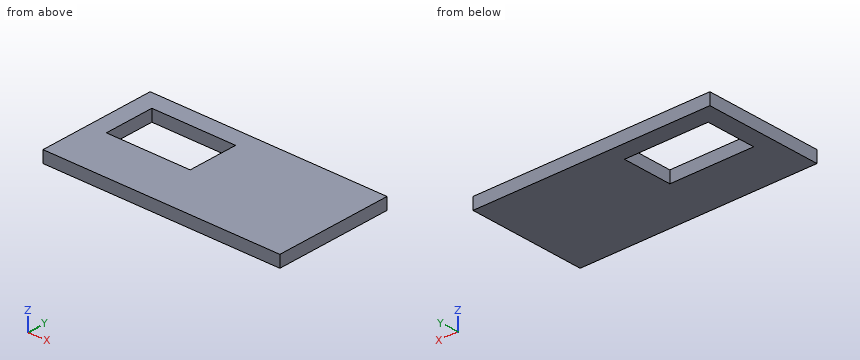
```python
from build123d import *

# Parameters (mm, degrees)
F0_W     = 200
F0_H     = 100
F1_DEPTH = 10
F3_DEPTH = 25


with BuildPart() as f1:
    # F0 (on Top) → F1 (new body)
    with BuildSketch(Plane.XY):
        with Locations((8.938173, -34.933871)):
            Rectangle(F0_W, F0_H)
    extrude(amount=F1_DEPTH)

    # F2 (on face) → F3 (cut)
    with BuildSketch(Plane.XY.offset(10)):
        Polygon((-5.306835, -42.385153), (-5.306835, 0), (-76.061827, 0.066129), (-76.061827, -42.385153), align=None)
    extrude(amount=-F3_DEPTH, mode=Mode.SUBTRACT)


solid = f1.part
```
Verification items for the finished model (mm, model axes). Give positions to 0.01 mm unless a question says otherwise; leave off trailing zeros. Order: outer loops, then holes, each group sorted by start corner. A loop starts at its lowest first (then second) coordinate and runs counter-clockwise, first axis right, second up. Notation, with made-up numbers: (43, -3.75) - (56, -3.75) arc R27 ccw to (56, 17.25) - close; hole circle Ø7 at (31, -35). An arc over 180 degrees is marked (long way). Answer as CSV lines item,"result". Start each with the question number.
Item 1: Section check C-C, the plane x = -46. Record the boundary of the cut face in (y, z).
Item 2: Material ranges on L1, parallel to X at y = -12, z = 8.25; L2, parallel to Y at x = -10, z = 4; L3, parallel to Y at x = -60.5, z = 4.5, recorded low to high.
Item 3: Section check A-A, the plane y = -39.5. Record the boundary of the cut face in (x, z), plus the area to 3 significant figures.
Item 4: Section check B-B, the plane z = 4.5. Record the boundary of the cut face in (x, y), plus the area to 3 significant figures.
Filled in:
1,outline,"(-84.93, 0) - (-42.39, 0) - (-42.39, 10) - (-84.93, 10) - close; (0.04, 0) - (15.07, 0) - (15.07, 10) - (0.04, 10) - close"
2,L1,"-91.06 to -76.06, -5.31 to 108.94"
2,L2,"-84.93 to -42.39, 0 to 15.07"
2,L3,"-84.93 to -42.39, 0.05 to 15.07"
3,outline,"(-91.06, 0) - (-76.06, 0) - (-76.06, 10) - (-91.06, 10) - close; (-5.31, 0) - (108.94, 0) - (108.94, 10) - (-5.31, 10) - close"
3,area,"1,290 mm^2"
4,outline,"(-91.06, -84.93) - (108.94, -84.93) - (108.94, 15.07) - (-91.06, 15.07) - close; hole (-76.06, -42.39) - (-5.31, -42.39) - (-5.31, 0) - (-76.06, 0.07) - close"
4,area,"17,000 mm^2"
